Work out the finished part from the listing and answer in its coordinate system (mm). A direction names the side the tool comes from. Coordinates: 2 decimals unless noted, no trailing zeros. Write each loop counter-clockwise with the first axis right and the second up, starting at its lowest first coordinate (ties: lowest second). Pieces come first, ordered by that corner, then holes. Notation, with made-up numbers: (22.25, 77) - (60.25, 77) arc R23 ccw to (60.25, 110) - close; hole circle Ø2 at (15, 51). An arc over 180 degrees is marked (long way). One line per item, written item: value.
```python
from build123d import *

# Parameters (mm, degrees)
SKETCH1_W                = 7
SKETCH1_H                = 40
BOSS_EXTRUDE1_DEPTH      = 50
BOSS_EXTRUDE2_DEPTH      = 4
BOSS_EXTRUDE2_DEPTH_BACK = 11
SKETCH3_W                = 40
SKETCH3_H                = 12.312299815
CHAMFER1_SIZE            = 7
FILLET1_R                = 4
SKETCH4_R                = 2
CUT_EXTRUDE2_DEPTH       = 10
SKETCH5_R                = 1.5
SKETCH5_R_2              = 2.75
CUT_EXTRUDE3_DEPTH       = 55.963624335
FILLET2_R                = 5
FILLET3_R                = 2


with BuildPart() as part:
    # Sketch1 → Boss-Extrude1 (new body)
    with BuildSketch(Plane(origin=(0, 0, 0), x_dir=(1, 0, 0), z_dir=(0, 1, 0))):
        Rectangle(SKETCH1_W, SKETCH1_H)
    extrude(amount=BOSS_EXTRUDE1_DEPTH)

    # Sketch3 → Boss-Extrude2 (add, two sides: drawn at the far end of the back side and taken through both)
    with BuildSketch(Plane(origin=(3.5, 0, 0), x_dir=(0, 0, -1), z_dir=(1, 0, 0)).offset(-BOSS_EXTRUDE2_DEPTH_BACK)):
        with Locations((0, 6.156149908)):
            Rectangle(SKETCH3_W, SKETCH3_H)
    extrude(amount=BOSS_EXTRUDE2_DEPTH + BOSS_EXTRUDE2_DEPTH_BACK)

    # Chamfer1
    # the kernel refuses this chamfer: 7 mm, written as the material it takes off along each edge
    with BuildSketch(Plane(origin=(-7.5, 12.312299815, 38.001780916), x_dir=(0.9996219169112968, 0.027495876610586365, 0), z_dir=(0, 0, -1))) as chamfer1_piece_1_section:
        Polygon((CHAMFER1_SIZE * 0.999621916911, CHAMFER1_SIZE * 0.0274958766106), (-CHAMFER1_SIZE * 0.0274958766106, CHAMFER1_SIZE * 0.999621916911), (0, 0), align=None)
    chamfer1_piece_1 = extrude(amount=76.003561832, mode=Mode.PRIVATE)
    chamfer1_piece_1 = split(chamfer1_piece_1, bisect_by=Plane(origin=(-3.5, 9.652025222, 0), z_dir=(-1, 0, 0)), keep=Keep.TOP, mode=Mode.PRIVATE)
    add(chamfer1_piece_1, mode=Mode.SUBTRACT)
    with BuildSketch(Plane(origin=(7.5, 12.312299815, 38.001780916), x_dir=(0.027495876610586365, -0.9996219169112968, 0), z_dir=(0, 0, -1))) as chamfer1_piece_2_section:
        Polygon((CHAMFER1_SIZE * 0.999621916911, CHAMFER1_SIZE * 0.0274958766106), (-CHAMFER1_SIZE * 0.0274958766106, CHAMFER1_SIZE * 0.999621916911), (0, 0), align=None)
    chamfer1_piece_2 = extrude(amount=76.003561832, mode=Mode.PRIVATE)
    chamfer1_piece_2 = split(chamfer1_piece_2, bisect_by=Plane(origin=(3.5, 9.652025222, 0), z_dir=(1, 0, 0)), keep=Keep.TOP, mode=Mode.PRIVATE)
    add(chamfer1_piece_2, mode=Mode.SUBTRACT)

    # Fillet1
    fillet1_edges = [part.edges().sort_by_distance(p)[0] for p in [
        (-7.5, 5.312299815, 0),
        (7.5, 5.312299815, 0),
        (-3.5, 9.312299815, 0),
        (3.5, 9.312299815, 0),
    ]]
    fillet(fillet1_edges, radius=FILLET1_R)

    # Sketch4 → Cut-Extrude2 (cut)
    with BuildSketch(Plane.XZ):
        with Locations(Location((0, 10, 0), (0, 0, 270))):
            Circle(SKETCH4_R)
        with Locations(Location((0, -10, 0), (0, 0, 90))):
            Circle(SKETCH4_R)
    extrude(amount=-CUT_EXTRUDE2_DEPTH, mode=Mode.SUBTRACT)

    # Sketch5 → Cut-Extrude3 (cut, through all)
    with BuildSketch(Plane.ZY.offset(3.5)):
        with Locations((-12.5, 30)):
            Circle(SKETCH5_R)
        with Locations((-6.25, 40.825317547)):
            Circle(SKETCH5_R)
        with Locations((6.25, 40.825317547)):
            Circle(SKETCH5_R)
        with Locations((12.5, 30)):
            Circle(SKETCH5_R)
        with Locations((6.25, 19.174682453)):
            Circle(SKETCH5_R)
        with Locations((-6.25, 19.174682453)):
            Circle(SKETCH5_R)
        with Locations((0, 30)):
            Circle(SKETCH5_R_2)
    extrude(amount=-CUT_EXTRUDE3_DEPTH, mode=Mode.SUBTRACT)

    # Fillet2
    fillet2_edges = [part.edges().sort_by_distance(p)[0] for p in [
        (0, 50, 20),
        (0, 50, -20),
    ]]
    fillet(fillet2_edges, radius=FILLET2_R)

    # Fillet3
    fillet3_edges = [part.edges().sort_by_distance(p)[0] for p in [
        (3.5, 50, 0),
        (-3.5, 50, 0),
        (-3.5, 27.984577032, -20),
        (-3.5, 27.984577032, 20),
        (-3.5, 48.535533906, 18.535533906),
        (-3.5, 48.535533906, -18.535533906),
        (3.5, 27.984577032, -20),
        (3.5, 27.984577032, 20),
        (3.5, 48.535533906, 18.535533906),
        (3.5, 48.535533906, -18.535533906),
        (-7.5, 1.827722783, -20),
        (7.5, 1.827722783, -20),
        (7.5, 1.827722783, 20),
        (-5.5, 7.312299815, 20),
        (-7.5, 1.827722783, 20),
        (5.5, 7.312299815, 20),
        (-7.19551813, 5.186179295, 20),
        (7.19551813, 5.186179295, 20),
        (5.5, 7.312299815, -20),
        (-5.5, 7.312299815, -20),
        (-7.19551813, 5.186179295, -20),
        (7.19551813, 5.186179295, -20),
        (-3.80448187, 9.438420335, 20),
        (-3.80448187, 9.438420335, -20),
        (3.80448187, 9.438420335, -20),
        (3.80448187, 9.438420335, 20),
    ]]
    fillet(fillet3_edges, radius=FILLET3_R)


solid = part.part
```
Item 1: Section C-C, the plane y = 22.5 is taken. Determine the outline of the cut face in (x, z).
Evaluation:
outline: (-3.5, -18) arc R2 ccw to (-1.5, -20) - (1.5, -20) arc R2 ccw to (3.5, -18) - (3.5, 18) arc R2 ccw to (1.5, 20) - (-1.5, 20) arc R2 ccw to (-3.5, 18) - close
Item 2: Determine the mould class of faces 1 (the face through (-5.1, 6.9, 19.4)), 2 (the face through (-0.05, 31.01, -13.61)), 3 (the face through (2.93, 27.75, -19.4)) for opening direction Y: +Y half, -Y half, draft (parallel to the pull), parting line (faces both ways), or undercut.
Evaluation:
face 1: +Y half
face 2: undercut
face 3: draft
Item 3: Given pin 1 (2 mm diameter, centred on x = -5.5, y = 13, fed in from +Z); pin 2 (18 mm diameter, centred on y = 20.5, z = 6, fed in from -X); pin 3 (5 mm diameter, centred on y = 30, z = -12.5, fed in from +X); pin 4 (1.2 mm diameter, centred on x = 0, z = 10, fed in from -Y), each flat-ended and moving along its own axis, determine where each tip first touches the part or whether it passes through.
Evaluation:
pin 1: passes through
pin 2: stops at x = -3.5
pin 3: stops at x = 3.5
pin 4: stops at y = 10
Item 4: Section B-B, the plane z = -1 is taken. Determine the outline of the cut face in (x, y).
Evaluation:
outline: (-7.5, 0) - (7.5, 0) - (7.5, 3.66) arc R4 ccw to (6.33, 6.48) - (4.67, 8.14) arc R4 cw to (3.5, 10.97) - (3.5, 27.44) - (-3.5, 27.44) - (-3.5, 10.97) arc R4 cw to (-4.67, 8.14) - (-6.33, 6.48) arc R4 ccw to (-7.5, 3.66) - close; (-3.5, 32.56) - (3.5, 32.56) - (3.5, 48) arc R2 ccw to (1.5, 50) - (-1.5, 50) arc R2 ccw to (-3.5, 48) - close
Item 5: Section A-A, the plane y = 30 is taken. Determine the outline of the cut face in (x, z), then the cut area to 3 significant figures.
Evaluation:
outline: (-3.5, -18) arc R2 ccw to (-1.5, -20) - (1.5, -20) arc R2 ccw to (3.5, -18) - (3.5, -14) - (-3.5, -14) - close; (-3.5, -11) - (3.5, -11) - (3.5, -2.75) - (-3.5, -2.75) - close; (-3.5, 2.75) - (3.5, 2.75) - (3.5, 11) - (-3.5, 11) - close; (-3.5, 14) - (3.5, 14) - (3.5, 18) arc R2 ccw to (1.5, 20) - (-1.5, 20) arc R2 ccw to (-3.5, 18) - close
area: 196 mm2
Item 6: Consider probe 1 along Y at (x, z) = (-1.25, 6.25); probe 2 along Z at (x, y) = (2.5, 41); probe 3 along Y at (x, z) = (-1, 0). Determine where each line is inside the solid, lowest interval first.
Evaluation:
probe 1: y = 0 to 17.67, 20.67 to 39.33, 42.33 to 50
probe 2: z = -19.73 to -7.74, -4.76 to 4.76, 7.74 to 19.73
probe 3: y = 0 to 27.25, 32.75 to 50
Item 7: Section D-D, the plane z = 6.25 is taken. Determine the outline of the cut face in (x, y).
Evaluation:
outline: (-7.5, 0) - (7.5, 0) - (7.5, 3.66) arc R4 ccw to (6.33, 6.48) - (4.67, 8.14) arc R4 cw to (3.5, 10.97) - (3.5, 17.67) - (-3.5, 17.67) - (-3.5, 10.97) arc R4 cw to (-4.67, 8.14) - (-6.33, 6.48) arc R4 ccw to (-7.5, 3.66) - close; (-3.5, 20.67) - (3.5, 20.67) - (3.5, 39.33) - (-3.5, 39.33) - close; (-3.5, 42.33) - (3.5, 42.33) - (3.5, 48) arc R2 ccw to (1.5, 50) - (-1.5, 50) arc R2 ccw to (-3.5, 48) - close
Item 8: Which of the six approach directions +Z, -Z, +X, -X, +Y, -Y give full straight-line access (tool end or side, diameter ignored) to faces 4 (the face through (6.93, 1.8, -19.4)), 5 (the face through (-3.5, 29, 4)), 6 (the face through (0, 10, 10))?
Evaluation:
face 4: -Z, +X, +Y, -Y
face 5: +Z, -Z, -X, +Y
face 6: -Y
